For this review, take the finished solid that the model builds, in its own axes (mm). A direction names the side the tool comes from. Give positions to 0.01 mm unless a question says otherwise; leave off trailing zeros. Write each loop counter-clockwise with the first axis right and the second up, starting at its lowest first coordinate (ties: lowest second). Pieces come first, ordered by that corner, then holes.
Autodesk Inventor part; units mm, degrees
ref_plane "YZ Plane" through (0, 0, 0) normal (1, 0, 0) x (0, 1, 0)
ref_plane "XZ Plane" through (0, 0, 0) normal (0, 1, 0) x (-1, 0, 0)
ref_plane "XY Plane" through (0, 0, 0) normal (0, 0, 1) x (1, 0, 0)
sketch "Skizze2" plane through (0, 0, 0) normal (0, 0, 1) x (1, 0, 0)
  line L0 (-177, 0) -> (177, 0)
  line L1 (177, 0) -> (177, 195)
  line L2 (177, 195) -> (-177, 195)
  line L3 (-177, 195) -> (-177, 0)
  point P0 (0, 0)
  point P1 (0, 0)
  dimension "d0" = 195
  dimension "d1" = 354
extrude "Extrusion1" add sketch "Skizze2" along normal blind 38
sketch "Skizze3" plane through (-177, 0, 0) normal (0, -1, 0) x (1, 0, 0)
  line L0 (354, 0) -> (0, 0)
  line L1 (0, 0) -> (15.5, 47)
  line L2 (15.5, 47) -> (0, 47)
  line L3 (0, 47) -> (0, 0)
  dimension "d7" = 15.5
extrude "Extrusion2" cut sketch "Skizze3" against normal up to surface (195 mm away)
mirror "Spiegeln1" about plane through (0, 0, 0) normal (1, 0, 0) of "Extrusion2"
fillet "Rundung1" radius 20 4 edges at (170.734, 0, 19) (170.734, 195, 19) (-170.734, 195, 19) (-170.734, 0, 19)
sketch "Skizze4" plane through (0, 0, 38) normal (0, 0, 1) x (1, 0, 0)
  ellipse E0 centre (-143.4086, 20) end of major axis (-164.4681, 20) minor radius 20 (-164.4681, 20) -> (-143.4086, 0) ccw
  line L0 (-143.4086, 0) -> (143.4086, 0)
  ellipse E1 centre (143.4086, 20) end of major axis (164.4681, 20) minor radius 20 (143.4086, 0) -> (164.4681, 20) ccw
  line L1 (164.4681, 20) -> (164.4681, 175)
  ellipse E2 centre (143.4086, 175) end of major axis (164.4681, 175) minor radius 20 (164.4681, 175) -> (143.4086, 195) ccw
  line L2 (143.4086, 195) -> (-143.4086, 195)
  ellipse E3 centre (-143.4086, 175) end of major axis (-164.4681, 175) minor radius 20 (-143.4086, 195) -> (-164.4681, 175) ccw
  line L3 (-164.4681, 175) -> (-164.4681, 20)
  line L4 (177, 60.5) -> (64, 60.5)
  line L5 (64, 60.5) -> (64, 85.5)
  line L6 (64, 85.5) -> (-116, 85.5)
  line L7 (-116, 85.5) -> (-116, 109.5)
  line L8 (-116, 109.5) -> (64, 109.5)
  line L9 (64, 109.5) -> (64, 134.5)
  line L10 (64, 134.5) -> (177, 134.5)
  line L11 (177, 20) -> (177, 175)
  line L12 (-177, 175) -> (-177, 20)
  line L13 (164.4681, 20) -> (164.4681, 175)
  point P0 (0, 0)
  point P1 (-116, 97.5)
  point P2 (164.4681, 97.5)
  point P3 (164.4681, 97.5)
  dimension "d12" = 113
  dimension "d14" = 24
  dimension "d15" = 74
  dimension "d16" = 37
  dimension "d17" = 180
extrude "Extrusion3" cut sketch "Skizze4" against normal blind 34 contours L4 L5 L6 L7 L8 L9 L10 L1 | L1 L10 L11 L4
sketch "Sketch7" plane through (64, 60.5, 38) normal (1, 0, 0) x (0, 0, -1)
  line L0 (0, 25) -> (34, 25)
  line L1 (34, 25) -> (34, 49)
  line L2 (0, 49) -> (34, 49)
  circle A0 centre (13, 37) radius 11
  line L3 (0, 25) -> (0, 49)
  point P0 (38, -60.5)
  point P1 (17, 49)
  point P2 (0, 37)
  dimension "d35" = 22
  dimension "d36" = 21
properties part number "1 part 1" material "Holz (Birke)"
(1) We need section C-C (x = 74.5). Write out the cut boundary in (y, z), and give its area (3 significant figures).
(2) Clearance check with flat-ended pins moving along their axes: pin 1 Ø7.5 at (y, z) = (71.5, 20.5) entering from +X; pin 2 Ø10 at (y, z) = (149.5, 7.5) entering from -X; pin 3 Ø8 at (x, y) = (86.5, 90) entering from +Z. State where each tip first meets the part, or that it passes through.
(3) The part is to be moulded in two halves that separate along Y. For faces 1 (the flat face through (121, 60.5, 21)), 2 (the flat face through (-116, 97, 21)), 3 (the flat face through (-2, 121, 38)), 4 (the flat face through (2, 195, 19)), say which applies: +Y half, -Y half, draft (parallel to the pull), parting line (faces both ways), or undercut.
(4) Tool access review of faces 5 (the flat face through (-2, 99, 0)), 6 (the flat face through (-27, 109.5, 21)): name each direction out of +Z, -Z, +X, -X, +Y, -Y from which nothing blocks a thin tool from reaching the whole face with its end or side.
(5) We need section B-B (y = 95). Write out the cut boundary in (x, z), and give its area (3 significant figures).
(6) We need section A-A (x = 32.5). Write out the cut boundary in (y, z).
(7) We need section D-D (y = 130.5). Write out the cut boundary in (x, z).
(8) For L1, parallel to Y at x = 46, z = 27; L2, parallel to Y at x = 107.5, z = 7; L3, parallel to Z at x = 32, y = 96, list the stretches that pass through material, from the lowest coordinate up.
The answers:
1. outline: (0, 0) - (195, 0) - (195, 38) - (134.5, 38) - (134.5, 4) - (60.5, 4) - (60.5, 38) - (0, 38) - close
1. area: 4,890 mm2
2. pin 1: stops at x = 64
2. pin 2: stops at x = -176.18
2. pin 3: stops at z = 4
3. face 1: undercut
3. face 2: undercut
3. face 3: draft
3. face 4: +Y half
4. face 5: -Z, +X, -X, +Y, -Y
4. face 6: +Z, +X
5. outline: (-177, 0) - (177, 0) - (175.68, 4) - (-116, 4) - (-116, 38) - (-164.47, 38) - close
5. area: 3,250 mm2
6. outline: (0, 0) - (195, 0) - (195, 38) - (109.5, 38) - (109.5, 4) - (85.5, 4) - (85.5, 38) - (0, 38) - close
7. outline: (-177, 0) - (177, 0) - (175.68, 4) - (64, 4) - (64, 38) - (-164.47, 38) - close
8. L1: y = 0 to 85.5, 109.5 to 195
8. L2: y = 0 to 60.5, 134.5 to 195
8. L3: z = 0 to 4
